Job drawing, mm, ordinate dimensions from the low corner. One solid piece. A direction names the side the tool comes from. Give positions to 0.01 mm unless a question says otherwise; leave off trailing zeros. Order: outer loops, then holes, each group sorted by start corner. A loop starts at its lowest first (then second) coordinate and runs counter-clockwise, first axis right, second up.
Item 1: Wall check: L1, parallel to Y at x = 16.5, z = 10.5; L2, parallel to X at y = 4.5, z = 9; L3, parallel to Z at x = 10.75, y = 4. Give the ranges that are in metal, low to high.
Item 2: Which spindle directions (+Z, -Z, +X, -X, +Y, -Y) get a long thin tool onto all of the face, cutting with end or side? Do the marked faces 1 and 2. Say none if no direction does.
Item 3: Flat gauge pins, fed straight in: P1, Ø2, axis at x = 7.5, y = 4.5, coming from the +Z side; P2, Ø1.5, axis at y = 1.5, z = 5, coming from the +X side; P3, Ø1.5, axis at x = 5, y = 5.5, coming from the -Z side. Where does each tip first touch, or does it go through?
Item 4: Band-saw the part on D-D on x = 15.5. Give the cut face in (y, z), plus the area to 3 significant figures.
Item 5: Band-saw the part on C-C on y = 3. Give the cut face in (x, z).
Item 6: Two-plate mould, pull along X, no slides. Class the marked faces 3, 4 and 5: released by +X, released by -X, zero draft, split by the parting line, or undercut.
Item 7: Band-saw the part on A-A on x = 9. Give the cut face in (y, z), plus the area to 3 significant figures.
Item 8: Band-saw the part on B-B on z = 9. Give the cut face in (x, y).
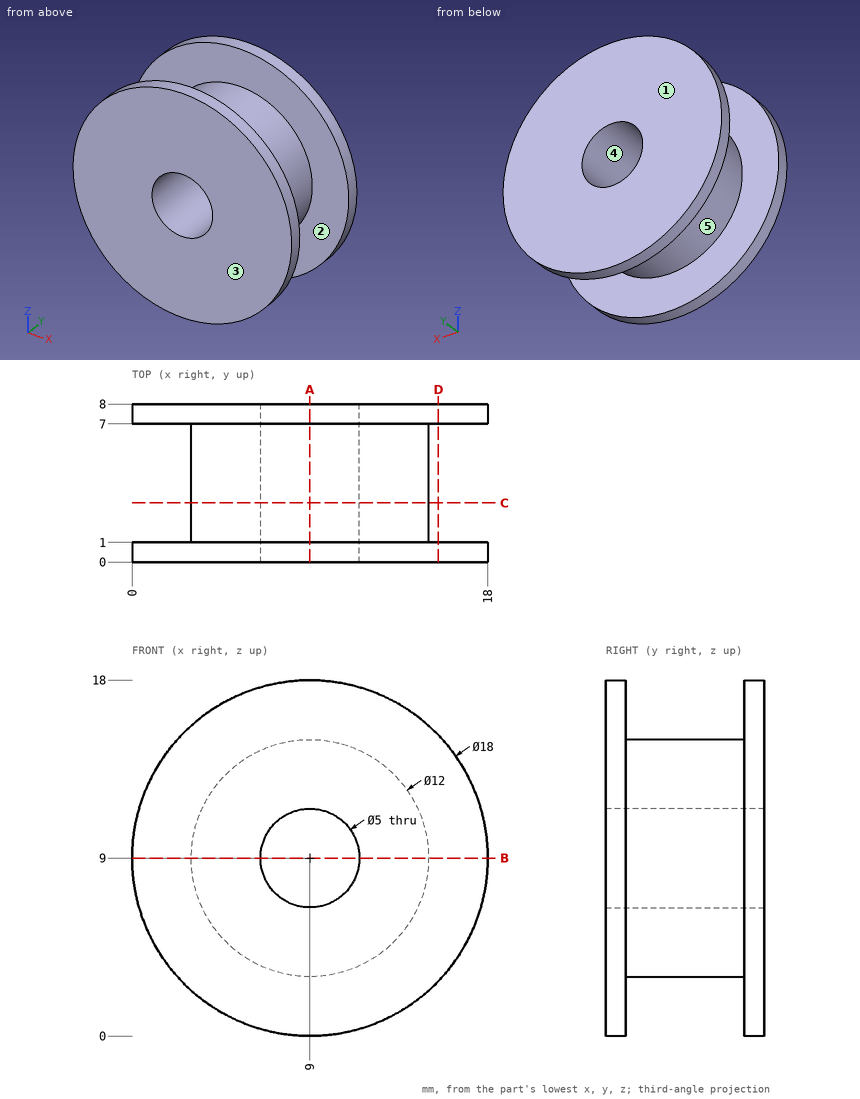
The answers:
1. L1: y = 0 to 1, 7 to 8
1. L2: x = 3 to 6.5, 11.5 to 15
1. L3: z = 3.26 to 7.21, 10.79 to 14.74
2. face 1: +Z, -Z, +X, -X, +Y
2. face 2: none
3. P1: stops at z = 14.98
3. P2: stops at x = 17.32
3. P3: stops at z = 3.96
4. outline: (0, 2.78) - (1, 2.78) - (1, 15.22) - (0, 15.22) - close; (7, 2.78) - (8, 2.78) - (8, 15.22) - (7, 15.22) - close
4. area: 24.9 mm2
5. outline: circle Ø12 at (9, 9); hole circle Ø5 at (9, 9)
6. face 3: zero draft
6. face 4: undercut
6. face 5: split by the parting line
7. outline: (0, 0) - (1, 0) - (1, 3) - (7, 3) - (7, 0) - (8, 0) - (8, 6.5) - (0, 6.5) - close; (0, 11.5) - (8, 11.5) - (8, 18) - (7, 18) - (7, 15) - (1, 15) - (1, 18) - (0, 18) - close
7. area: 68.0 mm2
8. outline: (0, 0) - (6.5, 0) - (6.5, 8) - (0, 8) - (0, 7) - (3, 7) - (3, 1) - (0, 1) - close; (11.5, 0) - (18, 0) - (18, 1) - (15, 1) - (15, 7) - (18, 7) - (18, 8) - (11.5, 8) - close
